```python
from build123d import *

# Parameters (mm, degrees)
SKIZZE1_R                                   = 29.925
AUFSATZ_LINEAR_AUSTRAGEN1_DEPTH             = 28
SCHNITT_LINEAR_AUSTRAGEN1_REACH             = 68.937
SKIZZE3_R                                   = 2.875
SCHNITT_LINEAR_AUSTRAGEN1_DIRECTION_2_DEPTH = 10
SKIZZE4_W                                   = 59.85
SKIZZE4_H                                   = 10
SCHNITT_LINEAR_AUSTRAGEN2_DEPTH             = 10
KREISMUSTER1_COUNT                          = 2
KREISMUSTER2_COUNT                          = 4
SKIZZE5_R                                   = 31.925
AUFSATZ_LINEAR_AUSTRAGEN2_DEPTH             = 0.8


with BuildPart() as part:
    # Skizze1 → Aufsatz-Linear austragen1 (new body)
    with BuildSketch(Plane(origin=(0, 0, 0), x_dir=(1, 0, 0), z_dir=(0, 1, 0))):
        with Locations(Location((0, 0, 0), (0, 0, 270))):
            Circle(SKIZZE1_R)
        with BuildLine():
            Line((-4, -20), (-20, -20))
            Line((-20, -20), (-20, -4))
            Line((-20, -4), (-15.4, -4))
            Line((-15.4, -4), (-15.4, -9.488825196))
            ThreePointArc((-15.4, -9.488825196), (-14.826178869, -10.347609207), (-13.813174058, -10.146110022))
            Line((-13.813174058, -10.146110022), (-8.12603127, -4.458967234))
            ThreePointArc((-8.12603127, -4.458967234), (-7.736711073, -3.876308384), (-7.6, -3.189015407))
            Line((-7.6, -3.189015407), (-7.6, 3.189015407))
            ThreePointArc((-7.6, 3.189015407), (-7.736711073, 3.876308384), (-8.12603127, 4.458967234))
            Line((-8.12603127, 4.458967234), (-13.813174058, 10.146110022))
            ThreePointArc((-13.813174058, 10.146110022), (-14.826178869, 10.347609207), (-15.4, 9.488825196))
            Line((-15.4, 9.488825196), (-15.4, 4))
            Line((-15.4, 4), (-20, 4))
            Line((-20, 4), (-20, 20))
            Line((-20, 20), (-4, 20))
            Line((-4, 20), (-4, 15.4))
            Line((-4, 15.4), (-9.488825196, 15.4))
            ThreePointArc((-9.488825196, 15.4), (-10.347609207, 14.826178869), (-10.146110022, 13.813174058))
            Line((-10.146110022, 13.813174058), (-4.458967234, 8.12603127))
            ThreePointArc((-4.458967234, 8.12603127), (-3.876308384, 7.736711073), (-3.189015407, 7.6))
            Line((-3.189015407, 7.6), (3.189015407, 7.6))
            ThreePointArc((3.189015407, 7.6), (3.876308384, 7.736711073), (4.458967234, 8.12603127))
            Line((4.458967234, 8.12603127), (10.146110022, 13.813174058))
            ThreePointArc((10.146110022, 13.813174058), (10.347609207, 14.826178869), (9.488825196, 15.4))
            Line((9.488825196, 15.4), (4, 15.4))
            Line((4, 15.4), (4, 20))
            Line((4, 20), (20, 20))
            Line((20, 20), (20, 4))
            Line((20, 4), (15.4, 4))
            Line((15.4, 4), (15.4, 9.488825196))
            ThreePointArc((15.4, 9.488825196), (14.826178869, 10.347609207), (13.813174058, 10.146110022))
            Line((13.813174058, 10.146110022), (8.12603127, 4.458967234))
            ThreePointArc((8.12603127, 4.458967234), (7.736711073, 3.876308384), (7.6, 3.189015407))
            Line((7.6, 3.189015407), (7.6, -3.189015407))
            ThreePointArc((7.6, -3.189015407), (7.736711073, -3.876308384), (8.12603127, -4.458967234))
            Line((8.12603127, -4.458967234), (13.813174058, -10.146110022))
            ThreePointArc((13.813174058, -10.146110022), (14.826178869, -10.347609207), (15.4, -9.488825196))
            Line((15.4, -9.488825196), (15.4, -4))
            Line((15.4, -4), (20, -4))
            Line((20, -4), (20, -20))
            Line((20, -20), (4, -20))
            Line((4, -20), (4, -15.4))
            Line((4, -15.4), (9.488825196, -15.4))
            ThreePointArc((9.488825196, -15.4), (10.347609207, -14.826178869), (10.146110022, -13.813174058))
            Line((10.146110022, -13.813174058), (4.458967234, -8.12603127))
            ThreePointArc((4.458967234, -8.12603127), (3.876308384, -7.736711073), (3.189015407, -7.6))
            Line((3.189015407, -7.6), (-3.189015407, -7.6))
            ThreePointArc((-3.189015407, -7.6), (-3.876308384, -7.736711073), (-4.458967234, -8.12603127))
            Line((-4.458967234, -8.12603127), (-10.146110022, -13.813174058))
            ThreePointArc((-10.146110022, -13.813174058), (-10.347609207, -14.826178869), (-9.488825196, -15.4))
            Line((-9.488825196, -15.4), (-4, -15.4))
            Line((-4, -15.4), (-4, -20))
        make_face(mode=Mode.SUBTRACT)
    extrude(amount=AUFSATZ_LINEAR_AUSTRAGEN1_DEPTH)

    # Skizze3 → Schnitt-Linear austragen1 (cut, up to next)
    with BuildSketch(Plane.ZY.offset(-23), mode=Mode.PRIVATE) as schnitt_linear_austragen1_sk1:
        with Locations((0, 23)):
            Circle(SKIZZE3_R)
    schnitt_linear_austragen1_tool1 = extrude(schnitt_linear_austragen1_sk1.sketch, amount=SCHNITT_LINEAR_AUSTRAGEN1_REACH, mode=Mode.PRIVATE) & part.part
    schnitt_linear_austragen1 = schnitt_linear_austragen1_tool1.solids().sort_by_distance((23, 23, 0))[0]
    add(schnitt_linear_austragen1, mode=Mode.SUBTRACT)

    # Skizze3 → Schnitt-Linear austragen1 direction 2 (cut)
    with BuildSketch(Plane.ZY.offset(-23)):
        with Locations((0, 23)):
            Circle(SKIZZE3_R)
    schnitt_linear_austragen1_direction_2 = extrude(amount=-SCHNITT_LINEAR_AUSTRAGEN1_DIRECTION_2_DEPTH, mode=Mode.SUBTRACT)

    # Skizze4 → Schnitt-Linear austragen2 (cut)
    with BuildSketch(Plane.ZY.offset(-23)):
        with Locations((0, 23)):
            Rectangle(SKIZZE4_W, SKIZZE4_H)
    schnitt_linear_austragen2 = extrude(amount=-SCHNITT_LINEAR_AUSTRAGEN2_DEPTH, mode=Mode.SUBTRACT)

    # Kreismuster1: Schnitt-Linear austragen1, Schnitt-Linear austragen1 direction 2 ×2 about axis
    kreismuster1_axis = Axis((0, 28, 0), (0, -1, 0))
    add([schnitt_linear_austragen1.rotate(kreismuster1_axis, i * 360 / KREISMUSTER1_COUNT) for i in range(1, KREISMUSTER1_COUNT)], mode=Mode.SUBTRACT)
    add([schnitt_linear_austragen1_direction_2.rotate(kreismuster1_axis, i * 360 / KREISMUSTER1_COUNT) for i in range(1, KREISMUSTER1_COUNT)], mode=Mode.SUBTRACT)

    # Kreismuster2: Schnitt-Linear austragen2 ×4 about axis
    kreismuster2_axis = Axis((0, 0, 0), (0, 1, 0))
    for i in range(1, KREISMUSTER2_COUNT):
        add(schnitt_linear_austragen2.rotate(kreismuster2_axis, i * 360 / KREISMUSTER2_COUNT), mode=Mode.SUBTRACT)

    # Skizze5 → Aufsatz-Linear austragen2 (add)
    with BuildSketch(Plane.XZ):
        with Locations(Location((0, 0, 0), (0, 0, 270))):
            Circle(SKIZZE5_R)
    extrude(amount=AUFSATZ_LINEAR_AUSTRAGEN2_DEPTH)


solid = part.part
```
Geometry: final body of the model. Coordinates: model frame, mm. Round coordinates to 2 decimals unless told otherwise and drop trailing zeros. Loops run counter-clockwise (first coordinate to the right, second up) from the corner with the lowest first, then second, coordinate; pieces in that order, holes last.
Item 1: Contact query for flat-ended pins moving along their axis: P1, Ø4.5, axis at y = 11.5, z = -8, coming from the +X side; P2, Ø1.5, axis at y = 17, z = 25.5, coming from the +X side; P3, Ø1.5, axis at x = 11, y = 18.5, coming from the -Z side. Output: stop coordinate, or through.
Checked values:
P1: stops at x = 29.37
P2: stops at x = 16.82
P3: stops at z = -28.04
Item 2: Section A-A, the plane z = 0. Output: boundary loops of the cut face in (x, y) (3 decimals), plus the area to 3 significant figures.
Checked values:
outline: (-31.925, -0.8) - (31.925, -0.8) - (31.925, 0) - (29.925, 0) - (29.925, 18) - (23, 18) - (23, 20.125) - (7.6, 20.125) - (7.6, 0) - (-7.6, 0) - (-7.6, 20.125) - (-23, 20.125) - (-23, 18) - (-29.925, 18) - (-29.925, 0) - (-31.925, 0) - close; (-23, 25.875) - (-7.6, 25.875) - (-7.6, 28) - (-23, 28) - close; (7.6, 25.875) - (23, 25.875) - (23, 28) - (7.6, 28) - close
area: 986 mm2
Item 3: Mould query, pull axis Y, two halves, no side actions, for faces 1 (the cylindrical face through (15.192, 20.193, -0.623)), 2 (the flat face through (26, 18, 0)), 3 (the cylindrical face through (-14.812, 13.804, -10.353)). Classes: released by +Y, released by -Y, zero draft, split by the parting line, or undercut.
Checked values:
face 1: undercut
face 2: released by +Y
face 3: zero draft
Item 4: Section B-B, the plane x = 0. Output: boundary loops of the cut face in (y, z) (3 decimals), plus the area to 3 significant figures.
Checked values:
outline: (-0.8, -31.925) - (0, -31.925) - (0, -29.925) - (18, -29.925) - (18, -23) - (28, -23) - (28, -7.6) - (0, -7.6) - (0, 7.6) - (28, 7.6) - (28, 23) - (18, 23) - (18, 29.925) - (0, 29.925) - (0, 31.925) - (-0.8, 31.925) - close
area: 1,160 mm2
Item 5: Line query: L1, parallel to X at y = 22, z = 16.5; L2, parallel to Z at x = 16.5, y = 23 (3 decimals); L3, parallel to Y at x = 14.25, z = 0 (3 decimals). Output: solid intervals per line, ascending.
Checked values:
L1: x = -23 to -20, -4 to 4, 20 to 23
L2: z = -23 to -20, -4 to -2.875, 2.875 to 4, 20 to 23
L3: y = -0.8 to 20.125, 25.875 to 28
Item 6: Section D-D, the plane z = 11.5. Output: boundary loops of the cut face in (x, y).
Checked values:
outline: (-29.78, -0.8) - (29.78, -0.8) - (29.78, 0) - (27.63, 0) - (27.63, 18) - (23, 18) - (23, 28) - (20, 28) - (20, 0) - (7.83, 0) - (7.83, 28) - (-7.83, 28) - (-7.83, 0) - (-20, 0) - (-20, 28) - (-23, 28) - (-23, 18) - (-27.63, 18) - (-27.63, 0) - (-29.78, 0) - close
Item 7: Section C-C, the plane x = -16.5. Output: boundary loops of the cut face in (y, z) (3 decimals), plus the area to 3 significant figures.
Checked values:
outline: (-0.8, -27.33) - (0, -27.33) - (0, -24.965) - (18, -24.965) - (18, -23) - (28, -23) - (28, -20) - (0, -20) - (0, -4) - (28, -4) - (28, 4) - (0, 4) - (0, 20) - (28, 20) - (28, 23) - (18, 23) - (18, 24.965) - (0, 24.965) - (0, 27.33) - (-0.8, 27.33) - close; hole circle Ø5.75 at (23, 0)
area: 481 mm2
